```python
from build123d import *

# Parameters (mm, degrees)
SKETCH1_R           = 1.7
SKETCH1_W           = 4
SKETCH1_H           = 3.175
SKETCH1_R_2         = 12
BOSS_EXTRUDE1_DEPTH = 3.175
SKETCH2_R           = 11.95936
SKETCH2_R_2         = 1.65936
SKETCH2_W           = 3.91872
SKETCH2_H           = 3.09372
BOSS_EXTRUDE2_DEPTH = 3.175


with BuildPart() as part:
    # Sketch1 → Boss-Extrude1 (new body)
    with BuildSketch(Plane.XY):
        Polygon((2, -33.175), (2, -30), (9.5, -30), (9.5, -33.175), (13.5, -33.175), (13.5, -30), (21.15, -30), (21.15, 30), (13.5, 30), (13.5, 33.175), (9.5, 33.175), (9.5, 30), (2, 30), (2, 33.175), (-2, 33.175), (-2, 30), (-9.5, 30), (-9.5, 33.175), (-13.5, 33.175), (-13.5, 30), (-21.15, 30), (-21.15, -30), (-13.5, -30), (-13.5, -33.175), (-9.5, -33.175), (-9.5, -30), (-2, -30), (-2, -33.175), align=None)
        with Locations((15.5, 15.5)):
            Circle(SKETCH1_R, mode=Mode.SUBTRACT)
        with Locations((-11.5, -25.9125)):
            Rectangle(SKETCH1_W, SKETCH1_H, mode=Mode.SUBTRACT)
        with Locations((0, -25.9125)):
            Rectangle(SKETCH1_W, SKETCH1_H, mode=Mode.SUBTRACT)
        with Locations((-15.5, -15.5)):
            Circle(SKETCH1_R, mode=Mode.SUBTRACT)
        with Locations((11.5, -25.9125)):
            Rectangle(SKETCH1_W, SKETCH1_H, mode=Mode.SUBTRACT)
        with Locations((15.5, -15.5)):
            Circle(SKETCH1_R, mode=Mode.SUBTRACT)
        with Locations((-15.5, 15.5)):
            Circle(SKETCH1_R, mode=Mode.SUBTRACT)
        Circle(SKETCH1_R_2, mode=Mode.SUBTRACT)
    extrude(amount=BOSS_EXTRUDE1_DEPTH)

    # Sketch2 → Boss-Extrude2 (add)
    with BuildSketch(Plane.XY.offset(3.175)):
        Polygon((-21.19064, 30.04064), (-21.19064, -30.04064), (-13.54064, -30.04064), (-13.54064, -33.21564), (-9.45936, -33.21564), (-9.45936, -30.04064), (-2.04064, -30.04064), (-2.04064, -33.21564), (2.04064, -33.21564), (2.04064, -30.04064), (9.45936, -30.04064), (9.45936, -33.21564), (13.54064, -33.21564), (13.54064, -30.04064), (21.19064, -30.04064), (21.19064, 30.04064), (13.54064, 30.04064), (13.54064, 33.21564), (9.45936, 33.21564), (9.45936, 30.04064), (2.04064, 30.04064), (2.04064, 33.21564), (-2.04064, 33.21564), (-2.04064, 30.04064), (-9.45936, 30.04064), (-9.45936, 33.21564), (-13.54064, 33.21564), (-13.54064, 30.04064), align=None)
        Circle(SKETCH2_R, mode=Mode.SUBTRACT)
        with Locations((-15.5, -15.5)):
            Circle(SKETCH2_R_2, mode=Mode.SUBTRACT)
        with Locations((15.5, -15.5)):
            Circle(SKETCH2_R_2, mode=Mode.SUBTRACT)
        with Locations((15.5, 15.5)):
            Circle(SKETCH2_R_2, mode=Mode.SUBTRACT)
        with Locations((-15.5, 15.5)):
            Circle(SKETCH2_R_2, mode=Mode.SUBTRACT)
        with Locations((11.5, -25.9125)):
            Rectangle(SKETCH2_W, SKETCH2_H, mode=Mode.SUBTRACT)
        with Locations((0, -25.9125)):
            Rectangle(SKETCH2_W, SKETCH2_H, mode=Mode.SUBTRACT)
        with Locations((-11.5, -25.9125)):
            Rectangle(SKETCH2_W, SKETCH2_H, mode=Mode.SUBTRACT)
    extrude(amount=-BOSS_EXTRUDE2_DEPTH)


solid = part.part
```
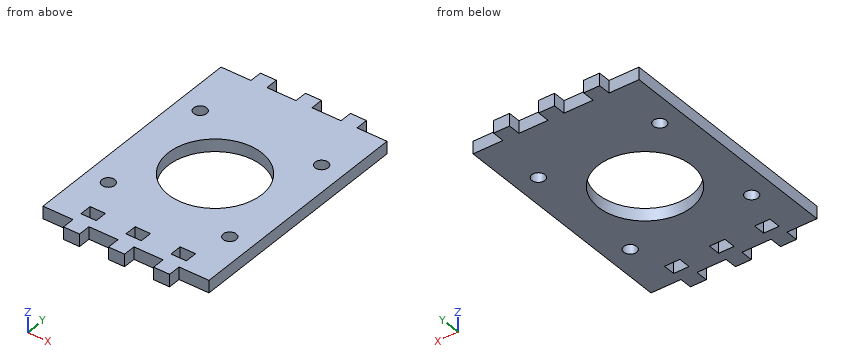
Geometry: final body of the model. Coordinates: model frame, mm. Round coordinates to 2 decimals unless told otherwise and drop trailing zeros. Order: outer loops, then holes, each group sorted by start corner. A loop starts at its lowest first (then second) coordinate and runs counter-clockwise, first axis right, second up. Notation, with made-up numbers: (38, 88.5) -> (76, 88.5) arc R26 ccw to (76, 126.5) -> close; hole circle Ø2 at (20.5, 89). An arc over 180 degrees is marked (long way). Write each question's results on one line, items separated by ' | '.
Q1. Section query D-D (z = 1.8). Count the separate pieces of the cut face and the enclosed holes in it, and give its area (3 significant figures).
Response values:
separate pieces: 1 | enclosed holes: 8 | area: 2,100 mm²
Q2. Ray query, line 1 along Y through (x, z) = (15.5, 2.25); line 2 along Y through (x, z) = (0, 1.05); line 3 along Y through (x, z) = (-12, 2.8). Return the intervals inside material, ascending.
Response values:
line 1: -30.04 to -17.16, -13.84 to 13.84, 17.16 to 30.04 | line 2: -33.22 to -27.46, -24.37 to -11.96, 11.96 to 33.22 | line 3: -33.22 to -27.46, -24.37 to 33.22
Q3. Section query B-B (y = 0). Output: boundary loops of the cut face in (x, z) (3 decimals), and give its area (3 significant figures).
Response values:
outline: (-21.191, 0) -> (-11.959, 0) -> (-11.959, 3.175) -> (-21.191, 3.175) -> close; (11.959, 0) -> (21.191, 0) -> (21.191, 3.175) -> (11.959, 3.175) -> close | area: 58.6 mm²
Q4. Pin query (flat end, axial travel): pin 1 Ø1 at (x, z) = (-4.5, 1) entering from -Y; pin 2 Ø1.5 at (x, z) = (4, 2) entering from +Y. Return the tip coordinate at first contact, or that it passes through.
Response values:
pin 1: y = -30.04 | pin 2: y = 30.04
Q5. Section query A-A (x = 0). Output: boundary loops of the cut face in (y, z) (3 decimals), and give its area (3 significant figures).
Response values:
outline: (-33.216, 0) -> (-27.459, 0) -> (-27.459, 3.175) -> (-33.216, 3.175) -> close; (-24.366, 0) -> (-11.959, 0) -> (-11.959, 3.175) -> (-24.366, 3.175) -> close; (11.959, 0) -> (33.216, 0) -> (33.216, 3.175) -> (11.959, 3.175) -> close | area: 125 mm²
Q6. Section query C-C (y = -15.5). Output: boundary loops of the cut face in (x, z) (3 decimals).
Response values:
outline: (-21.191, 0) -> (-17.159, 0) -> (-17.159, 3.175) -> (-21.191, 3.175) -> close; (-13.841, 0) -> (13.841, 0) -> (13.841, 3.175) -> (-13.841, 3.175) -> close; (17.159, 0) -> (21.191, 0) -> (21.191, 3.175) -> (17.159, 3.175) -> close
